Read the model definition and answer for the solid it produces. Units are mm, in the model's axes. A direction names the side the tool comes from. Coordinates: 2 decimals unless noted, no trailing zeros. Write each loop counter-clockwise with the first axis right and the second up, starting at its lowest first coordinate (ties: lowest second). Pieces come first, ordered by that corner, then holes. Notation, with made-up numbers: (68.5, 49) -> (76.5, 49) arc R26 cw to (76.5, 84) -> close; hole circle Ø11 at (0, 69.5). An arc over 180 degrees is marked (long way). Return JSON: item names as keys, results as strings.
Autodesk Inventor part; units mm, degrees
ref_plane "YZ Plane" through (0, 0, 0) normal (1, 0, 0) x (0, 1, 0)
ref_plane "XZ Plane" through (0, 0, 0) normal (0, 1, 0) x (-1, 0, 0)
ref_plane "XY Plane" through (0, 0, 0) normal (0, 0, 1) x (1, 0, 0)
sketch "Esboço1" plane through (0, 0, 0) normal (0, 0, 1) x (1, 0, 0)
  line L0 (-14, -9) -> (14, -9)
  line L1 (14, -9) -> (14, 9)
  line L2 (14, 9) -> (-14, 9)
  line L3 (-14, 9) -> (-14, -9)
  line L4 (-14, -9) -> (14, 9) construction
  line L5 (14, -9) -> (-14, 9) construction
  point P0 (0, 0)
  dimension "d0" = 18
  dimension "d3" = 28
extrude "Extrusão1" add sketch "Esboço1" along normal blind 29
sketch "Esboço2" plane through (0, 0, 29) normal (0, 0, 1) x (1, 0, 0)
  circle A0 centre (0, -1) radius 0.84
  line L0 (-14, -9) -> (14, -9)
  point P0 (0, 0)
  dimension "d4" = 1.68
  dimension "d5" = 8
extrude "Extrusão2" cut sketch "Esboço2" against normal blind 20
sketch "Esboço3" plane through (-14, -9, 0) normal (0, -1, 0) x (1, 0, 0)
  line L0 (8, 26.5) -> (20, 26.5)
  line L1 (20, 26.5) -> (20, 3.5)
  line L2 (20, 3.5) -> (8, 3.5)
  line L3 (8, 3.5) -> (8, 26.5)
  line L4 (0, 29) -> (28, 29)
  line L5 (0, 0) -> (28, 0)
  point P0 (14, 0)
  point P1 (14, 0)
  point P2 (14, 3.5)
  dimension "d8" = 2.5
  dimension "d9" = 12
  dimension "d10" = 0
  dimension "d11" = 23
extrude "Extrusão3" cut sketch "Esboço3" against normal blind 12
sketch "Esboço4" plane through (0, 0, 29) normal (0, 0, 1) x (1, 0, 0)
  line L0 (-14, 9) -> (-14, -9)
  line L1 (14, -9) -> (14, 9)
  point P0 (0, 0)
  point P1 (-10, 0)
  point P2 (10, 0)
  point P3 (-6, -9)
  point P4 (6, -9)
  dimension "d14" = 4
  dimension "d15" = 4
hole "Furo1" at (10, 0, 29) at (-10, 0, 29) direction (0, 0, -1) diameter 2.459 depth 16 tip angle 118
chamfer "Chanfro1" distance 3 angle 45 1 edges at (0, 9, 0)
fillet "Arredondamento1" radius 1 4 edges at (6, -3, 26.5) (-6, -3, 26.5) (-6, -3, 3.5) (6, -3, 3.5)
properties part number "CASE PROT IR" material "Poliacetal"
1. The part is cut by section D-D (z = 4). Determine the outline of the cut face in (x, y).
Taken from the geometry:
{"outline": "(-14, -9) -> (-5.87, -9) -> (-5.87, 3) -> (5.87, 3) -> (5.87, -9) -> (14, -9) -> (14, 9) -> (-14, 9) -> close"}
2. A tool of negligible diameter and unlimited length cuts with its end or side. For faces 4 (the face through (10.748, 0.976, 20.888)), 5 (the face through (14, 0, 14)), 6 (the face through (0, -3, 26.5)), from which of +Z, -Z, +X, -X, +Y, -Y can it reach the whole face along a straight path? Write none if from no direction.
Taken from the geometry:
{"face 4": "+Z", "face 5": "+Z, -Z, +X, +Y, -Y", "face 6": "-Y"}
3. For a pull along Y with two mould halves and no side action, classify faces 1 (the face through (10.064, -0.204, 12.39)), 2 (the face through (-6.4, -9, 14.3)), 3 (the face through (0, -1, 0)) as +Y half, -Y half, draft (parallel to the pull), parting line (faces both ways), or undercut.
Taken from the geometry:
{"face 1": "undercut", "face 2": "-Y half", "face 3": "draft"}
4. The part is cut by section B-B (x = 0). Determine the outline of the cut face in (y, z), then the cut area to 3 significant figures.
Taken from the geometry:
{"outline": "(-9, 0) -> (6, 0) -> (9, 3) -> (9, 29) -> (-0.16, 29) -> (-0.16, 26.5) -> (3, 26.5) -> (3, 3.5) -> (-9, 3.5) -> close; (-9, 26.5) -> (-1.84, 26.5) -> (-1.84, 29) -> (-9, 29) -> close", "area": "237 mm2"}
5. A flat-ended cylindrical pin translates along its axis: pin 1 Ø1.5 at (x, z) = (0, 4.5) entering from -Y. Find the tip coordinate at first contact, or state that the pin passes through.
Taken from the geometry:
{"pin 1": "stops at y = 3"}
6. The part is cut by section A-A (y = -6). Determine the outline of the cut face in (x, z).
Taken from the geometry:
{"outline": "(-14, 0) -> (14, 0) -> (14, 29) -> (-14, 29) -> close; hole (-6, 4.5) arc R1 ccw to (-5, 3.5) -> (5, 3.5) arc R1 ccw to (6, 4.5) -> (6, 25.5) arc R1 ccw to (5, 26.5) -> (-5, 26.5) arc R1 ccw to (-6, 25.5) -> close"}
7. Consider L1, parallel to X at y = 0, z = 18.75; L2, parallel to X at y = -8, z = 12.25; L3, parallel to Z at x = -1.5, y = -6.75. Determine where each line is inside the solid, lowest interval first.
Taken from the geometry:
{"L1": "x = -14 to -11.23, -8.77 to -6, 6 to 8.77, 11.23 to 14", "L2": "x = -14 to -6, 6 to 14", "L3": "z = 0 to 3.5, 26.5 to 29"}
8. The part is cut by section C-C (z = 15). Determine the outline of the cut face in (x, y), then the cut area to 3 significant figures.
Taken from the geometry:
{"outline": "(-14, -9) -> (-6, -9) -> (-6, 3) -> (6, 3) -> (6, -9) -> (14, -9) -> (14, 9) -> (-14, 9) -> close; hole circle Ø2.46 at (-10, 0); hole circle Ø2.46 at (10, 0)", "area": "351 mm2"}
